from build123d import *

# Parameters (mm, degrees)
SKETCH1_R                          = 25
SKETCH1_R_2                        = 4.8
BOSS_EXTRUDE1_DEPTH                = 3
F_4_0_4_DIAMETER_HOLE1_D           = 4
F_4_0_4_DIAMETER_HOLE1_CSINK_D     = 5
F_4_0_4_DIAMETER_HOLE1_CSINK_ANGLE = 90
FILLET2_R                          = 3


with BuildPart() as part:
    # Sketch1 → Boss-Extrude1 (new body)
    with BuildSketch(Plane(origin=(0, 0, 0), x_dir=(1, 0, 0), z_dir=(0, 1, 0))):
        with Locations(Location((0, 0, 0), (0, 0, 270))):
            Circle(SKETCH1_R)
        with Locations(Location((0, 0, 0), (0, 0, 270))):
            Circle(SKETCH1_R_2, mode=Mode.SUBTRACT)
    extrude(amount=BOSS_EXTRUDE1_DEPTH)

    # Ø4.0 (4) Diameter Hole1 (through all)
    with Locations(Plane(origin=(0, 3, 0), x_dir=(1, 0, 0), z_dir=(0, 1, 0))):
        with Locations((-7.5, 12.990381057), (15, 0), (-7.5, -12.990381057)):
            CounterSinkHole(F_4_0_4_DIAMETER_HOLE1_D / 2, F_4_0_4_DIAMETER_HOLE1_CSINK_D / 2, counter_sink_angle=F_4_0_4_DIAMETER_HOLE1_CSINK_ANGLE)

    # Sketch8 → Revolve1 (revolve)
    with BuildSketch(Plane.XY, mode=Mode.PRIVATE) as revolve1_sk:
        Polygon((27, 52), (29, 52), (6.8, 3), (4.8, 3), align=None)
    revolve(revolve1_sk.sketch.rotate(Axis((0, 0, 0), (0, 1, 0)), 270), axis=Axis((0, 0, 0), (0, 1, 0)))

    # Fillet2
    fillet2_edges = [part.edges().sort_by_distance(p)[0] for p in [
        (0, 3, -6.8),
    ]]
    fillet(fillet2_edges, radius=FILLET2_R)


solid = part.part
Input: part model. Units: mm. Frame: model coordinates. A direction names the side the tool comes from. Round coordinates to 2 decimals unless told otherwise and drop trailing zeros. Order: outer loops, then holes, each group sorted by start corner. A loop starts at its lowest first (then second) coordinate and runs counter-clockwise, first axis right, second up.
1. Cut plane A-A, the plane x = 0. Output: boundary loops of the cut face in (y, z), then the cut area to 3 significant figures.
The answers:
outline: (0, -25) - (3, -25) - (3, -11.45) arc R3 cw to (7.24, -8.72) - (52, -29) - (52, -27) - (3, -4.8) - (0, -4.8) - close; (0, 4.8) - (3, 4.8) - (52, 27) - (52, 29) - (7.24, 8.72) arc R3 cw to (3, 11.45) - (3, 25) - (0, 25) - close
area: 327 mm2
2. Cut plane C-C, the plane x = -7.5. State how many separate pieces and enclosed holes the cut face has, then the cut area to 3 significant figures.
The answers:
separate pieces: 3
enclosed holes: 0
area: 382 mm2
3. Cut plane D-D, the plane y = 18. Output: boundary loops of the cut face in (x, z), then the cut area to 3 significant figures.
The answers:
outline: circle Ø27.19 at (0, 0); hole circle Ø23.19 at (0, 0)
area: 158 mm2
4. Set-up query: faces 1 (the face through (4.05, 1.48, 2.58)), 2 (the face through (-11, 3, 5)), 3 (the face through (-7.24, 1.232, -14.973)). Return all of +Z, -Z, +X, -X, +Y, -Y with unobstructed straight access to the full face (end or side cutting, diameter ignored); none if empty.
The answers:
face 1: +Y, -Y
face 2: none
face 3: -Y
5. Pin query (flat end, axial travel): P1, Ø3, axis at x = -16, y = 46.5, coming from the +Z side; P2, Ø6, axis at x = 3, z = -20.5, coming from the +Y side; P3, Ø12, axis at y = 36, z = -18.5, coming from the -X side; P4, Ø1, axis at y = 7.5, z = 11, coming from the -X side. Return the tip coordinate at first contact, or that it passes through.
The answers:
P1: stops at z = 22.48
P2: stops at y = 44.76
P3: stops at x = -18.95
P4: passes through
6. Mould query, pull axis Z, two halves, no side actions, for faces 4 (the face through (4.082, 22.399, 12.961)), 5 (the face through (16.6, 1.2, 1.2)), 6 (the face through (-5, 0, 0)), 7 (the face through (-16.07, 24.33, -3.57)). Classes: released by +Z, released by -Z, zero draft, split by the parting line, or undercut.
The answers:
face 4: undercut
face 5: undercut
face 6: zero draft
face 7: split by the parting line
7. Material intervals for line 1 (Y direction, x = -8, z = 4); line 2 (X direction, y = 48.5, z = -1.5); line 3 (Y direction, x = 8, z = -4.5), sorted ascending.
The answers:
line 1: y = 0 to 4.35, 7.73 to 12.15
line 2: x = -27.37 to -25.37, 25.37 to 27.37
line 3: y = 0 to 4.04, 8.25 to 12.66
8. Cut plane B-B, the plane z = 0. Output: boundary loops of the cut face in (x, y).
The answers:
outline: (-29, 52) - (-8.72, 7.24) arc R3 cw to (-11.45, 3) - (-25, 3) - (-25, 0) - (-4.8, 0) - (-4.8, 3) - (-27, 52) - close; (4.8, 0) - (13, 0) - (13, 2.5) - (12.5, 3) - (11.45, 3) arc R3 cw to (8.72, 7.24) - (29, 52) - (27, 52) - (4.8, 3) - close; (17, 0) - (25, 0) - (25, 3) - (17.5, 3) - (17, 2.5) - close
